For this review, take the finished solid that the model builds, in its own axes (mm). Face numbers are marked on the shaded views. A direction names the side the tool comes from. Coordinates: 2 decimals unless noted, no trailing zeros. Loops run counter-clockwise (first coordinate to the right, second up) from the corner with the lowest first, then second, coordinate; pieces in that order, holes last. Notation, with made-up numbers: (69.25, 44) - (119.25, 44) arc R28 ccw to (119.25, 82) - close; hole circle Ø7 at (15, -16). An arc over 180 degrees is marked (long way). Answer as a JSON object with one key per item and string values. Group by question number.
Item 1: We need section C-C (z = 6.5). Give the boundary of the cut face in (x, y), then the cut area to 3 significant figures.
Item 2: To check wall thickness, follow line 1 (Z direction, x = 17.5, y = -7); line 2 (X direction, y = 9, z = 13.5); line 3 (X direction, y = 5.5, z = 27.5). State the ranges of each line that lie inside material, in increasing order.
Item 3: Tool access review of the marked faces 1, 2 and 3: name each direction out of +Z, -Z, +X, -X, +Y, -Y from which nothing blocks a thin tool from reaching the whole face with its end or side.
Item 4: Mouldability with a two-part tool opening along Y and no side actions: class the marked faces 4, 5, 6 and 7 as released by +Y, released by -Y, zero draft, split by the parting line, or undercut.
Item 5: We need section D-D (z = 22). Give the boundary of the cut face in (x, y).
Item 6: We need section B-B (y = -3). Give the boundary of the cut face in (x, z), then the cut area to 3 significant figures.
Item 7: We need section A-A (x = 42.5). Give the boundary of the cut face in (y, z), then the cut area to 3 significant figures.
Item 8: Clearance check with flat-ended pins moving along their axes: pin 1 (9.5 mm diameter, centred on x = 34.5, y = -1.5, fed in from -Z); pin 2 (8 mm diameter, centred on x = 23, y = -3, fed in from -Z); pin 3 (3 mm diameter, centred on x = 36, y = -2, fed in from +Z); pin 4 (6.5 mm diameter, centred on x = 33, z = 20, fed in from -Y). State where each tip first meets the part, or that it passes through.
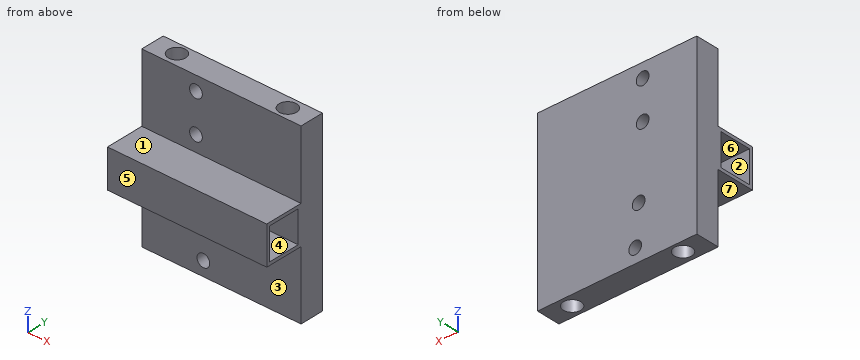
Autodesk Inventor part; units mm, degrees
ref_plane "Work Plane1" through (0, -9.0162, 2.2524) normal (0, 0, 1) x (1, 0, 0)
ref_plane "YZ Plane" through (0, 0, 0) normal (1, 0, 0) x (0, 1, 0)
ref_plane "XZ Plane" through (0, 0, 0) normal (0, 1, 0) x (-1, 0, 0)
sketch "Sketch1" plane through (0, 0, 0) normal (1, 0, 0) x (0, 1, 0)
  line L0 (2.9838, 8.2524) -> (-9.0162, 8.2524)
  line L1 (-9.0162, 8.2524) -> (-9.0162, -3.7476)
  line L2 (-9.0162, -3.7476) -> (2.9838, -3.7476)
  line L3 (2.9838, -3.7476) -> (2.9838, 8.2524)
  line L4 (1.9838, 7.2524) -> (-8.0162, 7.2524)
  line L5 (-8.0162, 7.2524) -> (-8.0162, -2.7476)
  line L6 (-8.0162, -2.7476) -> (1.9838, -2.7476)
  line L7 (1.9838, -2.7476) -> (1.9838, 7.2524)
  line L8 (10.4838, 29.7524) -> (2.9838, 29.7524)
  line L9 (2.9838, 29.7524) -> (2.9838, -25.2476)
  line L10 (2.9838, -25.2476) -> (10.4838, -25.2476)
  line L11 (10.4838, -25.2476) -> (10.4838, 29.7524)
  point P0 (0, 0)
  dimension "d0" = 12
  dimension "d1" = 10
  dimension "d2" = 10
  dimension "d3" = 12
  dimension "d4" = 1
  dimension "d5" = 1
  dimension "d22" = 21.5
  dimension "d24" = 55
  dimension "d25" = 7.5
  dimension "d55" = 21.5
extrude "Extrusion1" add sketch "Sketch1" along normal blind 50
ref_plane "Work Plane1" through (0, -9.0162, 2.2524) normal (0, 0, 1) x (1, 0, 0)
sketch "Sketch3" plane through (0, 2.9838, 29.7524) normal (0, 0, 1) x (1, 0, 0)
  line L0 (50, 7.5) -> (50, 0)
  line L1 (0, 7.5) -> (50, 7.5)
  point P0 (0, -2.9838)
  point P1 (7.5006, 3.9603)
  point P2 (42.5, 3.75)
  dimension "d26" = 35
  dimension "d27" = 7.5
  dimension "d28" = 50
  dimension "d29" = 7.5
  dimension "d30" = 3.75
hole "Hole1" at (42.5, 6.7338, 29.7524) at (7.5006, 6.944, 29.7524) direction (0, 0, -1) diameter 5.5 end through all
sketch "Sketch4" plane through (0, 10.4838, 29.7524) normal (0, 1, 0) x (1, 0, 0)
  line L0 (50, 55) -> (50, 0)
  line L1 (0, 0) -> (50, 0)
  line L2 (50, 21.5) -> (50, 33.5)
  line L3 (0, 55) -> (0, 0)
  line L4 (0, 55) -> (50, 55)
  point P0 (0, 29.7524)
  point P1 (17, 4.5)
  point P2 (17, 16.5)
  point P3 (19.3365, 50.5)
  point P4 (18.2576, 38.5)
  dimension "d38" = 33
  dimension "d39" = 4.5
  dimension "d40" = 12
  dimension "d57" = 12
  dimension "d58" = 4.5
hole "Hole3" at (19.3365, 10.4838, -20.7476) at (18.2576, 10.4838, -8.7476) at (17, 10.4838, 13.2524) at (17, 10.4838, 25.2524) direction (0, -1, 0) diameter 4 end through all
equation "\"d2\" = d1"
equation "\"d3\" = d0"
equation "\"d5\" = d4"
equation "\"d22\" = d55"
properties part number "fuselage_wing_interface"
Check sheet entries:
{
 "1": {"outline": "(0, -9.02) - (50, -9.02) - (50, -8.02) - (0, -8.02) - close; (0, 1.98) - (50, 1.98) - (50, 10.48) - (0, 10.48) - close; hole circle Ø5.5 at (7.5, 6.94); hole circle Ø5.5 at (42.5, 6.73)", "area": "427 mm2"},
 "2": {"line 1": "z = -3.75 to -2.75, 7.25 to 8.25", "line 2": "x = 0 to 5.67, 9.33 to 15.02, 18.98 to 40.94, 44.06 to 50", "line 3": "x = 0 to 5.16, 9.84 to 40.04, 44.96 to 50"},
 "3": {"face 1": "+Z, +X, -X, -Y", "face 2": "+X, -X", "face 3": "-Z, +X, -X, -Y"},
 "4": {"face 4": "undercut", "face 5": "released by -Y", "face 6": "undercut", "face 7": "zero draft"},
 "5": {"outline": "(0, 2.98) - (50, 2.98) - (50, 10.48) - (0, 10.48) - close; hole circle Ø5.5 at (7.5, 6.94); hole circle Ø5.5 at (42.5, 6.73)"},
 "6": {"outline": "(0, -3.75) - (50, -3.75) - (50, -2.75) - (0, -2.75) - close; (0, 7.25) - (50, 7.25) - (50, 8.25) - (0, 8.25) - close", "area": "100 mm2"},
 "7": {"outline": "(-9.02, -3.75) - (2.98, -3.75) - (2.98, -25.25) - (3.98, -25.25) - (3.98, 29.75) - (2.98, 29.75) - (2.98, 8.25) - (-9.02, 8.25) - close; (9.48, -25.25) - (10.48, -25.25) - (10.48, 29.75) - (9.48, 29.75) - close; hole (-8.02, -2.75) - (1.98, -2.75) - (1.98, 7.25) - (-8.02, 7.25) - close", "area": "154 mm2"},
 "8": {"pin 1": "stops at z = -25.25", "pin 2": "stops at z = -3.75", "pin 3": "stops at z = 8.25", "pin 4": "stops at y = 2.98"}
}
